from build123d import *

# Parameters (mm, degrees)
PAD_DEPTH       = 3.175
SKETCH001_R     = 8.0264
SKETCH001_R_2   = 4.7625
SKETCH001_R_3   = 2.46634
POCKET_DEPTH    = 3.176
FILLET_R        = 12.7
FILLET001_R     = 12.7
FILLET002_R     = 12.7
FILLET003_R     = 12.7
FILLET004_R     = 6.35
FILLET005_R     = 6.35
FILLET006_R     = 6.35
FILLET007_R     = 6.35
FILLET008_R     = 3.175
SKETCH002_R     = 2.2479
POCKET001_DEPTH = 3.176
FILLET009_R     = 6.35
FILLET010_R     = 6.35
FILLET011_R     = 3.175
FILLET012_R     = 3.175
SKETCH003_R     = 2.2479
POCKET002_DEPTH = 3.176


with BuildPart() as part:
    # Sketch → Pad (new body)
    with BuildSketch(Plane(origin=(-14.3421, 44.2432, 43.6758), x_dir=(1, 0, 0), z_dir=(0, 0, 1))):
        Polygon((37.363997, 35.9029), (-37.362803, 35.9029), (-37.362803, 88.9), (-56.412803, 88.9), (-130.912197, 12.700584), (-130.912197, -12.699416), (-56.413997, -88.9), (-37.363997, -88.9), (-37.363997, -35.9029), (37.362803, -35.9029), (37.362803, -88.9), (46.887803, -88.9), (46.887803, 88.9), (37.363997, 88.9), align=None)
    extrude(amount=PAD_DEPTH)

    # Sketch001 → Pocket (cut, through all)
    with BuildSketch(Plane(origin=(-14.3421, 44.2432, 46.8508), x_dir=(1, 0, 0), z_dir=(0, 0, 1))):
        with Locations((-69.533135, 42.978666)):
            Circle(SKETCH001_R)
        with Locations((-118.212197, 0.000584)):
            Circle(SKETCH001_R_2)
        with Locations((-18.211203, 29.5529)):
            Circle(SKETCH001_R_3)
        with Locations((18.212397, 29.5529)):
            Circle(SKETCH001_R_3)
        with Locations((-18.211203, 16.8529)):
            Circle(SKETCH001_R_3)
        with Locations((18.212397, 16.8529)):
            Circle(SKETCH001_R_3)
        with Locations((-18.211203, -16.8529)):
            Circle(SKETCH001_R_3)
        with Locations((18.212397, -16.8529)):
            Circle(SKETCH001_R_3)
        with Locations((-18.211203, -29.5529)):
            Circle(SKETCH001_R_3)
        with Locations((18.212397, -29.5529)):
            Circle(SKETCH001_R_3)
    extrude(amount=-POCKET_DEPTH, mode=Mode.SUBTRACT)

    # Fillet
    fillet_edges = [part.edges().sort_by_distance(p)[0] for p in [
        (-145.254297, 56.943784, 45.2633),
    ]]
    fillet(fillet_edges, radius=FILLET_R)

    # Fillet001
    fillet001_edges = [part.edges().sort_by_distance(p)[0] for p in [
        (-145.254297, 31.543784, 45.2633),
    ]]
    fillet(fillet001_edges, radius=FILLET001_R)

    # Fillet002
    fillet002_edges = [part.edges().sort_by_distance(p)[0] for p in [
        (-70.756097, -44.6568, 45.2633),
    ]]
    fillet(fillet002_edges, radius=FILLET002_R)

    # Fillet003
    fillet003_edges = [part.edges().sort_by_distance(p)[0] for p in [
        (-70.754903, 133.1432, 45.2633),
    ]]
    fillet(fillet003_edges, radius=FILLET003_R)

    # Fillet004
    fillet004_edges = [part.edges().sort_by_distance(p)[0] for p in [
        (-51.706097, -44.6568, 45.2633),
    ]]
    fillet(fillet004_edges, radius=FILLET004_R)

    # Fillet005
    fillet005_edges = [part.edges().sort_by_distance(p)[0] for p in [
        (-51.704903, 133.1432, 45.2633),
    ]]
    fillet(fillet005_edges, radius=FILLET005_R)

    # Fillet006
    fillet006_edges = [part.edges().sort_by_distance(p)[0] for p in [
        (-51.706097, 8.3403, 45.2633),
    ]]
    fillet(fillet006_edges, radius=FILLET006_R)

    # Fillet007
    fillet007_edges = [part.edges().sort_by_distance(p)[0] for p in [
        (23.020703, 8.3403, 45.2633),
    ]]
    fillet(fillet007_edges, radius=FILLET007_R)

    # Fillet008
    fillet008_edges = [part.edges().sort_by_distance(p)[0] for p in [
        (23.020703, -44.6568, 45.2633),
    ]]
    fillet(fillet008_edges, radius=FILLET008_R)

    # Sketch002 → Pocket001 (cut, through all)
    with BuildSketch(Plane(origin=(-14.3421, 44.2432, 46.8508), x_dir=(1, 0, 0), z_dir=(0, 0, 1))):
        with Locations((-63.581526, 75.195872)):
            Circle(SKETCH002_R)
        with Locations((-86.246322, 52.96145)):
            Circle(SKETCH002_R)
        with Locations((-86.247007, -52.960923)):
            Circle(SKETCH002_R)
        with Locations((-63.582545, -75.195686)):
            Circle(SKETCH002_R)
    extrude(amount=-POCKET001_DEPTH, mode=Mode.SUBTRACT)

    # Fillet009
    fillet009_edges = [part.edges().sort_by_distance(p)[0] for p in [
        (-51.704903, 80.1461, 45.2633),
    ]]
    fillet(fillet009_edges, radius=FILLET009_R)

    # Fillet010
    fillet010_edges = [part.edges().sort_by_distance(p)[0] for p in [
        (23.021897, 80.1461, 45.2633),
    ]]
    fillet(fillet010_edges, radius=FILLET010_R)

    # Fillet011
    fillet011_edges = [part.edges().sort_by_distance(p)[0] for p in [
        (23.021897, 133.1432, 45.2633),
        (32.545703, 133.1432, 45.2633),
    ]]
    fillet(fillet011_edges, radius=FILLET011_R)

    # Fillet012
    fillet012_edges = [part.edges().sort_by_distance(p)[0] for p in [
        (32.545703, -44.6568, 45.2633),
    ]]
    fillet(fillet012_edges, radius=FILLET012_R)

    # Sketch003 → Pocket002 (cut, through all)
    with BuildSketch(Plane(origin=(-14.3421, 44.2432, 46.8508), x_dir=(1, 0, 0), z_dir=(0, 0, 1))):
        with Locations((42.125303, -28.575)):
            Circle(SKETCH003_R)
        with Locations((42.125303, 79.375)):
            Circle(SKETCH003_R)
        with Locations((42.125303, -79.375)):
            Circle(SKETCH003_R)
        with Locations((42.125303, 28.575)):
            Circle(SKETCH003_R)
    extrude(amount=-POCKET002_DEPTH, mode=Mode.SUBTRACT)


solid = part.part
Read the model definition and answer for the solid it produces. Units are mm, in the model's axes. A direction names the side the tool comes from. Coordinates: 2 decimals unless noted, no trailing zeros. Write each loop counter-clockwise with the first axis right and the second up, starting at its lowest first coordinate (ties: lowest second). Pieces come first, ordered by that corner, then holes. Notation, with made-up numbers: (-24, -22) -> (34, -22) arc R18 ccw to (34, 5) -> close; hole circle Ø11 at (67, 80.5). An arc over 180 degrees is marked (long way). Return JSON: item names as keys, results as strings.
(1) For a pull along Y with two mould halves and no side action, classify faces 4 (the cylindrical face through (3.549, 17.136, 45.286)), 5 (the cylindrical face through (-128.01, 45.67, 45.29)), 6 (the cylindrical face through (-70.403, -43.635, 45.286)), 7 (the cylindrical face through (-49.8, 81.96, 45.29)) as pulls with the +Y half, pulls with the -Y half, needs draft (parallel to the pull), parting line crosses it, or undercut.
Answers below:
{"face 4": "undercut", "face 5": "undercut", "face 6": "pulls with the -Y half", "face 7": "pulls with the +Y half"}
(2) The part is cut by section A-A on x = -84.5. Give the vertices of the cut face in (y, z).
Answers below:
{"outline": "(-30.6, 43.68) -> (79.22, 43.68) -> (79.22, 46.85) -> (-30.6, 46.85) -> close; (95.22, 43.68) -> (119.08, 43.68) -> (119.08, 46.85) -> (95.22, 46.85) -> close"}
(3) The part is cut by section B-B on y = -15. Give the vertices of the cut face in (x, z).
Answers below:
{"outline": "(-99.75, 43.68) -> (-51.71, 43.68) -> (-51.71, 46.85) -> (-99.75, 46.85) -> close; (23.02, 43.68) -> (32.55, 43.68) -> (32.55, 46.85) -> (23.02, 46.85) -> close"}
(4) Which of the six approach directions +Z, -Z, +X, -X, +Y, -Y give full straight-line access (tool end or side, diameter ignored) to faces 1 (the cylindrical face through (-98.445, -8.043, 45.286)), 2 (the cylindrical face through (-53.62, -42.85, 45.29)), 3 (the cylindrical face through (21.112, 81.957, 45.286))?
Answers below:
{"face 1": "+Z, -Z", "face 2": "+Z, -Z, -Y", "face 3": "+Z, -Z, +Y"}
(5) The part is cut by section C-C on x = -20.5. Give the vertices of the cut face in (y, z).
Answers below:
{"outline": "(8.34, 43.68) -> (80.15, 43.68) -> (80.15, 46.85) -> (8.34, 46.85) -> close"}
(6) Each of these flat-tipped pins is pushed along its axis until it touches: P1, Ø1.6, axis at x = -6, z = 45.5, coming from the +Y side; P2, Ø1.5, axis at x = -119, y = 84.5, coming from the -Z side; P3, Ø1, axis at y = 85.5, z = 46.5, coming from the -X side. Where does it stop, or does it pass through?
Answers below:
{"P1": "y = 80.15", "P2": "z = 43.68", "P3": "x = -117.82"}
(7) The part is cut by section D-D on z = 46.2. State how many separate pieces and enclosed holes the cut face has, then the cut area to 3 significant figures.
Answers below:
{"separate pieces": "1", "enclosed holes": "18", "area": "17,500 mm^2"}
(8) Consider line 1 along X through (y, z) = (92.5, 45.75); line 2 along X through (y, z) = (-10, 46.05); line 3 along Y through (x, z) = (-100.5, 44.6). Determine where each line is inside the solid, lowest interval first. Write a range as from..to.
Answers below:
{"line 1": "-110.49..-89.92, -77.83..-51.7, 23.02..32.55", "line 2": "-104.64..-102.44, -98.74..-51.71, 23.02..32.55", "line 3": "-14.23..-10.96, -6.47..94.96, 99.45..102.72"}
